from build123d import *

# Parameters (mm, degrees)
SKETCH1_W           = 25
SKETCH1_H           = 70
BOSS_EXTRUDE1_DEPTH = 15
CUT_EXTRUDE1_REACH  = 74.672
SKETCH2_W           = 21
SKETCH2_H           = 13
SKETCH4_W           = 25
SKETCH4_H           = 15
SKETCH4_W_2         = 7.320869851
SKETCH4_H_2         = 3.892108022
BOSS_EXTRUDE2_DEPTH = 3
CUT_EXTRUDE3_REACH  = 41.373
SKETCH5_R           = 3.6


with BuildPart() as part:
    # Sketch1 → Boss-Extrude1 (new body)
    with BuildSketch(Plane.XY):
        Rectangle(SKETCH1_W, SKETCH1_H)
    extrude(amount=-BOSS_EXTRUDE1_DEPTH)

    # Sketch2 → Cut-Extrude1 (cut, up to next)
    with BuildSketch(Plane(origin=(0, 35, 0), x_dir=(1, 0, 0), z_dir=(0, 1, 0)), mode=Mode.PRIVATE) as cut_extrude1_sk1:
        with Locations((0, 8.5)):
            Rectangle(SKETCH2_W, SKETCH2_H)
    cut_extrude1_tool1 = extrude(cut_extrude1_sk1.sketch, amount=-CUT_EXTRUDE1_REACH, mode=Mode.PRIVATE) & part.part
    add(cut_extrude1_tool1.solids().sort_by_distance((0, 35, -8.5))[0], mode=Mode.SUBTRACT)

    # Sketch4 → Boss-Extrude2 (add)
    with BuildSketch(Plane(origin=(0, 35, 0), x_dir=(1, 0, 0), z_dir=(0, 1, 0))):
        with Locations((0, 7.5)):
            Rectangle(SKETCH4_W, SKETCH4_H)
        with Locations((0.092669239, 5.540570559)):
            Rectangle(SKETCH4_W_2, SKETCH4_H_2, mode=Mode.SUBTRACT)
    extrude(amount=-BOSS_EXTRUDE2_DEPTH)

    # Sketch5 → Cut-Extrude3 (cut, up to next)
    with BuildSketch(Plane(origin=(0, 0, -2), x_dir=(-1, 0, 0), z_dir=(0, 0, -1)), mode=Mode.PRIVATE) as cut_extrude3_sk1:
        with Locations((0, 20)):
            Circle(SKETCH5_R)
    cut_extrude3_tool1 = extrude(cut_extrude3_sk1.sketch, amount=-CUT_EXTRUDE3_REACH, mode=Mode.PRIVATE) & part.part
    # Sketch5 → Cut-Extrude3 (cut, up to next)
    with BuildSketch(Plane(origin=(0, 0, -2), x_dir=(-1, 0, 0), z_dir=(0, 0, -1)), mode=Mode.PRIVATE) as cut_extrude3_sk2:
        with Locations((0, -25)):
            Circle(SKETCH5_R)
    cut_extrude3_tool2 = extrude(cut_extrude3_sk2.sketch, amount=-CUT_EXTRUDE3_REACH, mode=Mode.PRIVATE) & part.part
    add(cut_extrude3_tool1.solids().sort_by_distance((0, 20, -2))[0], mode=Mode.SUBTRACT)
    add(cut_extrude3_tool2.solids().sort_by_distance((0, -25, -2))[0], mode=Mode.SUBTRACT)


solid = part.part
Geometry: final body of the model. Coordinates: model frame, mm. A direction names the side the tool comes from. Give positions to 0.01 mm unless a question says otherwise; leave off trailing zeros. Write each loop counter-clockwise with the first axis right and the second up, starting at its lowest first coordinate (ties: lowest second). Pieces come first, ordered by that corner, then holes. Notation, with made-up numbers: (62, -35.75) -> (121, -35.75) arc R29 cw to (121, -2.75) -> close; hole circle Ø8 at (86, 69). An arc over 180 degrees is marked (long way). Answer as a JSON object with one key per item and string values.
1. Ray query, probe 1 along Y at (x, z) = (0, -1.15); probe 2 along X at (y, z) = (29, -8); probe 3 along Y at (x, z) = (6, -6.25). Return the intervals inside material, ascending. Write a range as from..to.
Ans:
{"probe 1": "y = -35..-28.6, -21.4..16.4, 23.6..35", "probe 2": "x = -12.5..-10.5, 10.5..12.5", "probe 3": "y = 32..35"}
2. Cut plane D-D on z = -9.25. Output: boundary loops of the cut face in (x, y).
Ans:
{"outline": "(-12.5, -35) -> (-10.5, -35) -> (-10.5, 32) -> (10.5, 32) -> (10.5, -35) -> (12.5, -35) -> (12.5, 35) -> (-12.5, 35) -> close"}
3. Mould query, pull axis Z, two halves, no side actions, for faces 1 (the flat face through (0, 0, 0)), 2 (the flat face through (-2, -35, -1)), 3 (the flat face through (-3.568, 34, -6)). Classes: pulls with the +Z half, pulls with the -Z half, needs draft (parallel to the pull), parting line crosses it, or undercut.
Ans:
{"face 1": "pulls with the +Z half", "face 2": "needs draft", "face 3": "undercut"}
4. Cut plane A-A on z = -6. Output: boundary loops of the cut face in (x, y).
Ans:
{"outline": "(-12.5, -35) -> (-10.5, -35) -> (-10.5, 32) -> (-3.57, 32) -> (-3.57, 35) -> (-12.5, 35) -> close; (3.75, 32) -> (10.5, 32) -> (10.5, -35) -> (12.5, -35) -> (12.5, 35) -> (3.75, 35) -> close"}
5. Contact query for a flat-ended pin moving along its axis: pin 1 (8 mm diameter, centred on x = -3, z = -7.5, fed in from -Y). Output: stop coordinate, or through.
Ans:
{"pin 1": "stops at y = 32"}
6. Access query for faces 4 (the flat face through (0, 35, -9)), 5 (the flat face through (0, 32, -9)), 6 (the flat face through (0, 34, -3.595)). Directions: +Z, -Z, +X, -X, +Y, -Y. A direction counts if a zero-diameter tool reaches every point of the face in a straight line with its end or side. Return the directions, or none.
Ans:
{"face 4": "+Z, -Z, +X, -X, +Y", "face 5": "-Z, -Y", "face 6": "+Y, -Y"}
7. Cut plane B-B on y = 20. Output: boundary loops of the cut face in (x, z), and give its area (3 significant figures).
Ans:
{"outline": "(-12.5, -15) -> (-10.5, -15) -> (-10.5, -2) -> (-3.6, -2) -> (-3.6, 0) -> (-12.5, 0) -> close; (3.6, -2) -> (10.5, -2) -> (10.5, -15) -> (12.5, -15) -> (12.5, 0) -> (3.6, 0) -> close", "area": "87.6 mm^2"}
8. Cut plane C-C on x = 0. Output: boundary loops of the cut face in (y, z), and give its area (3 significant figures).
Ans:
{"outline": "(-35, -2) -> (-28.6, -2) -> (-28.6, 0) -> (-35, 0) -> close; (-21.4, -2) -> (16.4, -2) -> (16.4, 0) -> (-21.4, 0) -> close; (23.6, -2) -> (32, -2) -> (32, -3.59) -> (35, -3.59) -> (35, 0) -> (23.6, 0) -> close; (32, -15) -> (35, -15) -> (35, -7.49) -> (32, -7.49) -> close", "area": "139 mm^2"}
